Autodesk Inventor part; units mm, degrees
ref_plane "YZ Plane" through (0, 0, 0) normal (1, 0, 0) x (0, 1, 0)
ref_plane "XZ Plane" through (0, 0, 0) normal (0, 1, 0) x (-1, 0, 0)
ref_plane "XY Plane" through (0, 0, 0) normal (0, 0, 1) x (1, 0, 0)
sketch "Sketch1" plane through (0, 0, 0) normal (0, 0, 1) x (1, 0, 0)
  arc A0 (0, -146.05) -> (0, 146.05) centre (0, 0) ccw
  line L0 (0, 0) -> (0, 226.0912) construction
  line L1 (0, 226.0912) -> (0, -237.3269) construction
  line L2 (6.35, 145.9119) -> (6.35, 171.3324)
  line L3 (6.35, -145.9119) -> (6.35, -171.3324)
  line L4 (0, 146.05) -> (0, 151.13)
  line L5 (0, 151.13) -> (6.35, 151.13)
  line L6 (6.35, 151.13) -> (-7.62, 151.13)
  line L7 (-7.62, 151.13) -> (-7.62, 161.29)
  line L8 (-7.62, 161.29) -> (6.35, 161.29)
  line L9 (0, -146.05) -> (0, -151.13)
  line L10 (0, -151.13) -> (6.35, -151.13)
  line L11 (6.35, -151.13) -> (-7.62, -151.13)
  line L12 (-7.62, -151.13) -> (-7.62, -161.29)
  line L13 (-7.62, -161.29) -> (6.35, -161.29)
  line L14 (171.45, 0) -> (171.45, -69.85)
  line L15 (171.45, -69.85) -> (156.5761, -69.85)
  arc A1 (0, -171.45) -> (156.5761, -69.85) centre (0, 0) ccw
  arc A2 (171.45, 0) -> (0, 171.45) centre (0, 0) ccw
  dimension "d20" = 292.1
  dimension "d21" = 6.35
  dimension "d22" = 6.35
  dimension "d23" = 5.08
  dimension "d24" = 13.97
  dimension "d25" = 10.16
  dimension "d26" = 5.08
  dimension "d27" = 13.97
  dimension "d28" = 10.16
  dimension "d29" = 69.85
  dimension "d45" = 171.45
  dimension "d46" = 171.45
extrude "Extrusion5" add sketch "Sketch1" along normal blind 6.35 contours A0 L2 A2 L14 L15 A1 L3 | L10 L3 L13 L12 L11 | L5 L6 L7 L8 L2
sketch "Sketch3" plane through (0, 0, 6.35) normal (0, 0, 1) x (1, 0, 0)
  arc A0 (6.35, -171.3324) -> (156.5761, -69.85) centre (0, 0) ccw
  line L0 (156.5761, -69.85) -> (171.45, -69.85)
  line L1 (171.45, -69.85) -> (171.45, 0)
  arc A1 (171.45, 0) -> (6.35, 171.3324) centre (0, 0) ccw
  line L2 (6.35, 171.3324) -> (6.35, 161.29)
  line L3 (154.305, -22.1996) -> (154.305, -32.3596)
  line L4 (154.305, -32.3596) -> (163.83, -32.3596)
  line L5 (163.83, -32.3596) -> (163.83, -22.1996)
  line L6 (163.83, -22.1996) -> (154.305, -22.1996)
  line L7 (154.305, -15.1718) -> (171.45, -15.1718)
  line L8 (171.45, 0) -> (171.45, -15.1718)
  line L9 (154.305, -15.1718) -> (154.305, -10.0918)
  line L10 (154.305, -10.0918) -> (171.45, 0)
  line L11 (171.45, -69.85) -> (171.45, -44.45)
  line L12 (171.45, -44.45) -> (154.305, -44.45)
  line L13 (154.305, -44.45) -> (154.305, -74.7333)
  dimension "d53" = 10.16
  dimension "d54" = 9.525
  dimension "d55" = 10.16
  dimension "d56" = 37.4904
  dimension "d57" = 7.62
  dimension "d58" = 17.145
  dimension "d59" = 5.08
  dimension "d60" = 25.4
extrude "Extrusion7" cut sketch "Sketch3" against normal blind 25.4
sketch "Sketch4" plane through (0, 0, 6.35) normal (0, 0, 1) x (1, 0, 0)
  line L0 (6.35, -161.29) -> (6.35, -171.3324)
  arc A0 (6.35, -171.3324) -> (154.305, -74.7333) centre (0, 0) ccw
  line L1 (33.4395, -168.1574) -> (6.35, -168.1574)
  dimension "d63" = 3.175
extrude "Extrusion8" cut sketch "Sketch4" against normal blind 25.4
properties part number "MiddleHoop"
Could you check a few things on this model? Use its own coordinates, in mm. A direction names the side the tool comes from. Coordinates: 2 decimals unless noted, no trailing zeros. Order: outer loops, then holes, each group sorted by start corner. A loop starts at its lowest first (then second) coordinate and runs counter-clockwise, first axis right, second up. Notation, with made-up numbers: M -6,-20 L 17,-20 A25 cw 17,0 Z; hole C 29,-2 d9. An arc over 180 degrees is marked long. Use one line per item in the form item = value. Start each with the question number.
1. For pin 1 (3 mm diameter, centred on x = 13, z = 1.5, fed in from +Y); pin 2 (1.5 mm diameter, centred on y = -13.5, z = 1.5, fed in from +X) (3 decimals); pin 3 (1.5 mm diameter, centred on y = -35.5, z = 3, fed in from -X), each with a flat end and sliding along its axis, tell me the tip position at first contact or that it passes through.
2. Suppose I cut it at C-C on y = 4.5. Write out the boundary of the cut face in (x, z).
3. Suppose I cut it at B-B on z = 1. Write out the boundary of the cut face in (x, y) (3 decimals).
4. We'd pull the mould along X, two halves only. Please class faces 1 (the flat face through (-1, -151.13, 3)), 2 (the flat face through (159, -32.36, 3)), 3 (the flat face through (-7.62, -156, 3)), 4 (the flat face through (163.83, -27, 3)): +X half, -X half, draft (parallel to the pull), parting line (faces both ways), or undercut.
5. On a 3-axis mill with a long thin cutter (end or side, diameter ignored), from which of +Z, -Z, +X, -X, +Y, -Y can I reach the whole of each face in a straight line? I mean faces 5 (the flat face through (-1, -161.29, 3)), 6 (the flat face through (-1, 161.29, 3)), 7 (the flat face through (154.305, -59, 3)). Say none if no direction works.
6. Suppose I cut it at A-A on x = 0. Write out the boundary of the cut face in (y, z), then the cut area to 3 significant figures.
7. Please list where these lines run through material, in increasing order: line 1 (Y direction, x = 81.5, z = 2.5); line 2 (Y direction, x = 114.5, z = 1.75); line 3 (X direction, y = 2, z = 5).
8. Suppose I cut it at D-D on x = 54. Write out the boundary of the cut face in (y, z), then the cut area to 3 significant figures.
Geometry says:
q1.pin_1 = 171.06
q1.pin_2 = 154.305
q1.pin_3 = 141.48
q2.outline = M 145.98,0 L 171.39,0 L 171.39,6.35 L 145.98,6.35 Z
q3.outline = M -7.62,-161.29 L 6.35,-161.29 L 6.35,-168.157 L 33.439,-168.157 A171.45 ccw 154.305,-74.733 L 154.305,-44.45 L 171.45,-44.45 L 171.45,-15.172 L 154.305,-15.172 L 154.305,-10.092 L 171.45,0 A171.45 ccw 6.35,171.332 L 6.35,161.29 L -7.62,161.29 L -7.62,151.13 L 6.35,151.13 L 6.35,145.912 A146.05 cw 6.35,-145.912 L 6.35,-151.13 L -7.62,-151.13 Z; hole M 154.305,-32.36 L 163.83,-32.36 L 163.83,-22.2 L 154.305,-22.2 Z
q4.face_1 = draft
q4.face_2 = undercut
q4.face_3 = -X half
q4.face_4 = undercut
q5.face_5 = +Z, -Z, -X, -Y
q5.face_6 = +Z, -Z, -X, +Y
q5.face_7 = +Z, -Z, +X, -Y
q6.outline = M -161.29,0 L -151.13,0 L -151.13,6.35 L -161.29,6.35 Z; M 151.13,0 L 161.29,0 L 161.29,6.35 L 151.13,6.35 Z
q6.area = 129 mm^2
q7.line_1 = -150.84 to -121.2, 121.2 to 150.84
q7.line_2 = -127.61 to -90.67, 90.67 to 127.61
q7.line_3 = 146.04 to 171.44
q8.outline = M -162.72,0 L -135.7,0 L -135.7,6.35 L -162.72,6.35 Z; M 135.7,0 L 162.72,0 L 162.72,6.35 L 135.7,6.35 Z
q8.area = 343 mm^2
